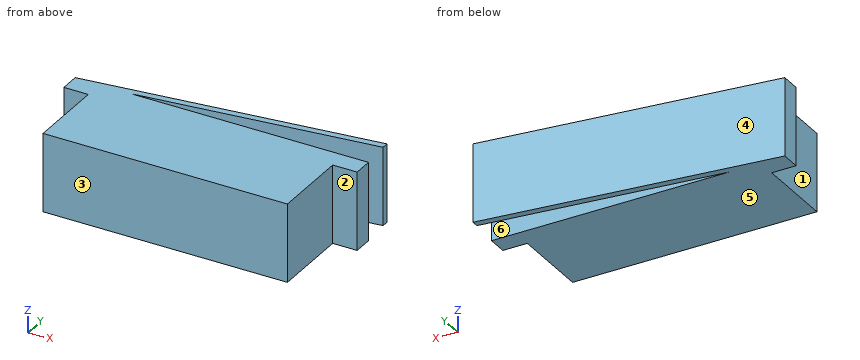
```python
from build123d import *

# Parameters (mm, degrees)
SKETCH1_W           = 25
SKETCH1_H           = 8
BOSS_EXTRUDE1_DEPTH = 8


with BuildPart() as part:
    # Sketch1 → Boss-Extrude1 (new body)
    with BuildSketch(Plane.XY):
        Polygon((14.776384549, 9.656080302), (-15, 6), (-9.346191937, 6), (14.776384549, 8.961879962), align=None)
        Polygon((-9.346191937, 6), (-15, 6), (-15, 4), (-12.5, 4), (12.5, 4), (15, 4), (15, 6), align=None)
        Rectangle(SKETCH1_W, SKETCH1_H)
    extrude(amount=BOSS_EXTRUDE1_DEPTH)


solid = part.part
```
The listing builds one solid part. Answer for the finished solid, in the listing's coordinates (mm). Face numbers are marked on the shaded views. A direction names the side the tool comes from. Coordinates: 2 decimals unless noted, no trailing zeros. Write each loop counter-clockwise with the first axis right and the second up, starting at its lowest first coordinate (ties: lowest second). Pieces come first, ordered by that corner, then holes. Notation, with made-up numbers: (68, -12) - (103, -12) arc R11 cw to (103, 3) - close; hole circle Ø7 at (20.5, 6.5). An arc over 180 degrees is marked (long way). Return JSON: item names as keys, results as strings. Group by question number.
Q1. The part is cut by section A-A on x = -0.75. Write down the section's boundary in (y, z), and give its area (3 significant figures).
Q2. The part is cut by section D-D on x = -11.25. Write down the section's boundary in (y, z).
Q3. For a pull along Y with two mould halves and no side action, classify the marked faces 4, 5 and 6 as +Y half, -Y half, draft (parallel to the pull), parting line (faces both ways), or undercut.
Q4. Which of the six approach directions +Z, -Z, +X, -X, +Y, -Y give full straight-line access (tool end or side, diameter ignored) to the marked faces 1, 2 and 3?
Q5. Flat-ended cylindrical pins translate along their axes: pin 1 Ø0.8 at (y, z) = (9.5, 2.5) entering from +X; pin 2 Ø2.5 at (x, z) = (5, 3.5) entering from +Y; pin 3 Ø0.8 at (x, z) = (14, 5) entering from -Y. Find the tip coordinate at first contact, or state that the pin passes through.
Q6. Find the intervals of material crossed by line 1 along X through (y, z) = (-1.25, 2); line 2 along Y through (x, z) = (-5.5, 7); line 3 along Y through (x, z) = (-1.25, 7.75), in increasing order. Write a range as [from, to].
Q7. The part is cut by section C-C on y = 1.25. Write down the section's boundary in (x, z), and give its area (3 significant figures).
Q8. The part is cut by section B-B on z = 2.5. Write down the section's boundary in (x, y).
Evaluation:
{
 "1": {"outline": "(-4, 0) - (6, 0) - (6, 8) - (-4, 8) - close; (7.06, 0) - (7.75, 0) - (7.75, 8) - (7.06, 8) - close", "area": "85.6 mm2"},
 "2": {"outline": "(-4, 0) - (6.46, 0) - (6.46, 8) - (-4, 8) - close"},
 "3": {"face 4": "+Y half", "face 5": "draft", "face 6": "undercut"},
 "4": {"face 1": "+Z, -Z, -X, -Y", "face 2": "+Z, -Z, +X, -Y", "face 3": "+Z, -Z, +X, -X, -Y"},
 "5": {"pin 1": "stops at x = 14.78", "pin 2": "stops at y = 8.61", "pin 3": "stops at y = 4"},
 "6": {"line 1": "x = [-12.5, 12.5]", "line 2": "y = [-4, 6], [6.47, 7.17]", "line 3": "y = [-4, 6], [6.99, 7.69]"},
 "7": {"outline": "(-12.5, 0) - (12.5, 0) - (12.5, 8) - (-12.5, 8) - close", "area": "200 mm2"},
 "8": {"outline": "(-15, 4) - (-12.5, 4) - (-12.5, -4) - (12.5, -4) - (12.5, 4) - (15, 4) - (15, 6) - (-9.35, 6) - (14.78, 8.96) - (14.78, 9.66) - (-15, 6) - close"}
}
